Design review of the part built by this model. Coordinates are the model's own, in mm. Face numbers are marked on the shaded views. A direction names the side the tool comes from. Coordinates: 2 decimals unless noted, no trailing zeros. Write each loop counter-clockwise with the first axis right and the second up, starting at its lowest first coordinate (ties: lowest second). Pieces come first, ordered by that corner, then holes. Notation, with made-up numbers: (42.25, -8) -> (90.25, -8) arc R30 ccw to (90.25, 22) -> close; hole circle Ø4 at (32.5, -35). An arc over 180 degrees is marked (long way). Answer in a Markdown table with one row per item. Add a question column.
Item 1: Take a section at B-B, the plane x = 7.5. Write out the cut boundary in (y, z) (3 decimals).
Item 2: Draft analysis for pull direction X (two halves, no side actions). For the marked faces 1, 2 and 3, state which applies: released by +X, released by -X, zero draft, split by the parting line, or undercut.
Item 3: To check wall thickness, follow line 1 (X direction, y = 115.5, z = 21) (3 decimals); line 2 (Y direction, x = 25, z = 50). State the ranges of each line that lie inside material, in increasing order.
Item 4: Take a section at A-A, the plane z = 30. Write out the cut boundary in (x, y) (3 decimals).
Item 5: Clearance check with a flat-ended pin moving along its axis: P1, Ø6, axis at x = 7, z = 20, coming from the -Y side. State where the tip first meets the part, or that it passes through.
Item 6: For the marked faces 4 and 5, list the 3-axis set-ups (+Z, -Z, +X, -X, +Y, -Y) from which the entire face can be reached by the end or side of a thin tool; tool diameter is ignored.
Item 7: Take a section at C-C, the plane y = 232. Write out the cut boundary in (x, z) (3 decimals).
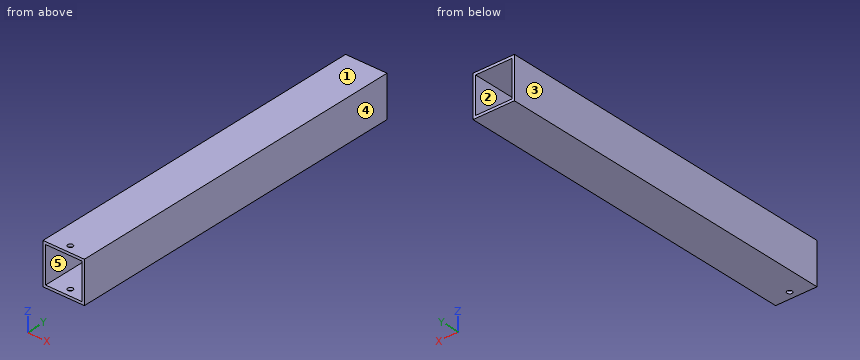
Autodesk Inventor part; units mm, degrees
ref_plane "YZ Plane" through (0, 0, 0) normal (1, 0, 0) x (0, 1, 0)
ref_plane "XZ Plane" through (0, 0, 0) normal (0, 1, 0) x (-1, 0, 0)
ref_plane "XY Plane" through (0, 0, 0) normal (0, 0, 1) x (1, 0, 0)
sketch "Sketch1" plane through (0, 0, 0) normal (0, 0, 1) x (1, 0, 0)
  line L0 (0, 0) -> (50.8, 0)
  line L1 (50.8, 0) -> (50.8, 431.8)
  line L2 (50.8, 431.8) -> (0, 431.8)
  line L3 (0, 431.8) -> (0, 0)
  dimension "d0" = 50.8
  dimension "d1" = 431.8
extrude "Extrusion1" add sketch "Sketch1" along normal blind 50.8
shell "Shell1" thickness 3.175 removed faces 2 at (33.8667, 431.8, 16.9333) at (16.9333, 0, 16.9333)
sketch "Sketch3" plane through (0, 0, 50.8) normal (0, 0, 1) x (1, 0, 0)
  line L0 (50.8, 0) -> (0, 0)
  line L1 (50.8, 431.8) -> (50.8, 0)
  circle A0 centre (25.4, 9.525) radius 3.175
  dimension "d10" = 9.525
  dimension "d11" = 25.4
  dimension "d12" = 6.35
extrude "Extrusion3" cut sketch "Sketch3" against normal through all
properties part number "CentralColumn" material "Aluminum-6061"
Answers:
| question | item | result |
|---|---|---|
| 1 | outline | (0, 0) -> (431.8, 0) -> (431.8, 3.175) -> (0, 3.175) -> close; (0, 47.625) -> (431.8, 47.625) -> (431.8, 50.8) -> (0, 50.8) -> close |
| 2 | face 1 | zero draft |
| 2 | face 2 | undercut |
| 2 | face 3 | released by -X |
| 3 | line 1 | x = 0 to 3.175, 47.625 to 50.8 |
| 3 | line 2 | y = 0 to 6.38, 12.67 to 431.8 |
| 4 | outline | (0, 0) -> (3.175, 0) -> (3.175, 431.8) -> (0, 431.8) -> close; (47.625, 0) -> (50.8, 0) -> (50.8, 431.8) -> (47.625, 431.8) -> close |
| 5 | P1 | passes through |
| 6 | face 4 | +Z, -Z, +X, +Y, -Y |
| 6 | face 5 | +Y, -Y |
| 7 | outline | (0, 0) -> (50.8, 0) -> (50.8, 50.8) -> (0, 50.8) -> close; hole (3.175, 3.175) -> (47.625, 3.175) -> (47.625, 47.625) -> (3.175, 47.625) -> close |
